Job drawing, mm, ordinate dimensions from the low corner. One solid piece. Round coordinates to 2 decimals unless told otherwise and drop trailing zeros. Loops run counter-clockwise (first coordinate to the right, second up) from the corner with the lowest first, then second, coordinate; pieces in that order, holes last. Notation, with made-up numbers: M 8.5,31 L 52.5,31 A21 ccw 52.5,47 Z; hole C 74,24 d4. An arc over 180 degrees is marked long. One line per item, written item: value.
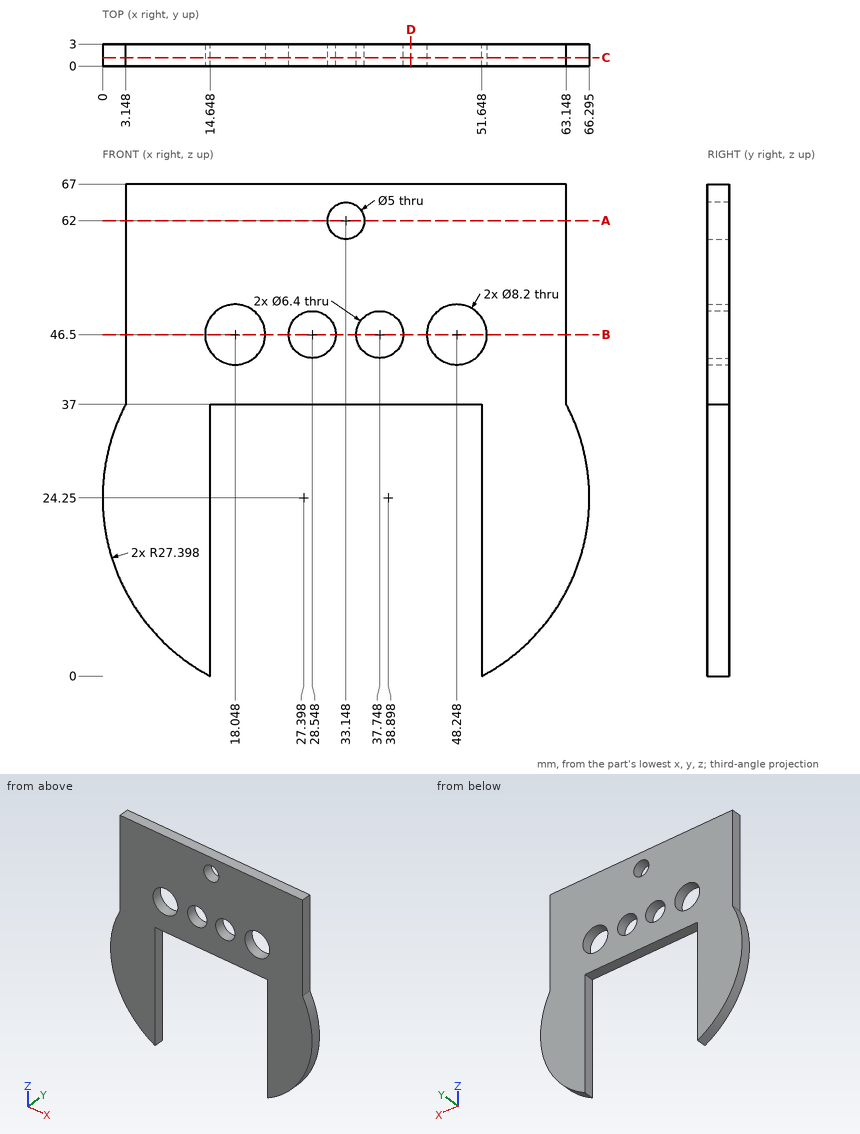
Item 1: Slice it at C-C, the plane y = 1.15. Give the number of separate pieces and of enclosed holes in the cut face, and give its area (3 significant figures).
Check values:
separate pieces: 1
enclosed holes: 5
area: 2,460 mm2
Item 2: Slice it at D-D, the plane x = 42. Give the cut face in (y, z).
Check values:
outline: M 0,37 L 3,37 L 3,67 L 0,67 Z
Item 3: Slice it at A-A, the plane z = 62. Give the cut face in (x, y).
Check values:
outline: M 3.15,0 L 30.65,0 L 30.65,3 L 3.15,3 Z; M 35.65,0 L 63.15,0 L 63.15,3 L 35.65,3 Z
Item 4: Slice it at B-B, the plane z = 46.5. Give the cut face in (x, y).
Check values:
outline: M 3.15,0 L 13.95,0 L 13.95,3 L 3.15,3 Z; M 22.15,0 L 25.35,0 L 25.35,3 L 22.15,3 Z; M 31.75,0 L 34.55,0 L 34.55,3 L 31.75,3 Z; M 40.95,0 L 44.15,0 L 44.15,3 L 40.95,3 Z; M 52.35,0 L 63.15,0 L 63.15,3 L 52.35,3 Z
Item 5: Wall check: line 1 along X through (y, z) = (1.6, 46.5); line 2 along X through (y, z) = (1.15, 62); line 3 along X through (y, z) = (2.1, 45.5) (1 decimal). Give the ranges that are in metal, low to high.
Check values:
line 1: x = 3.15 to 13.95, 22.15 to 25.35, 31.75 to 34.55, 40.95 to 44.15, 52.35 to 63.15
line 2: x = 3.15 to 30.65, 35.65 to 63.15
line 3: x = 3.1 to 14.1, 22 to 25.5, 31.6 to 34.7, 40.8 to 44.3, 52.2 to 63.1
Item 6: Drop flat-ended pins along their axis: P1, Ø0.9, axis at y = 2, z = 20, coming from the +X side; P2, Ø1, axis at y = 2.5, z = 20, coming from the -X side; P3, Ø1.5, axis at y = 1.5, z = 58, coming from the +X side. Give the stop position or say it passes through.
Check values:
P1: stops at x = 66.03
P2: stops at x = 0.26
P3: stops at x = 63.15
